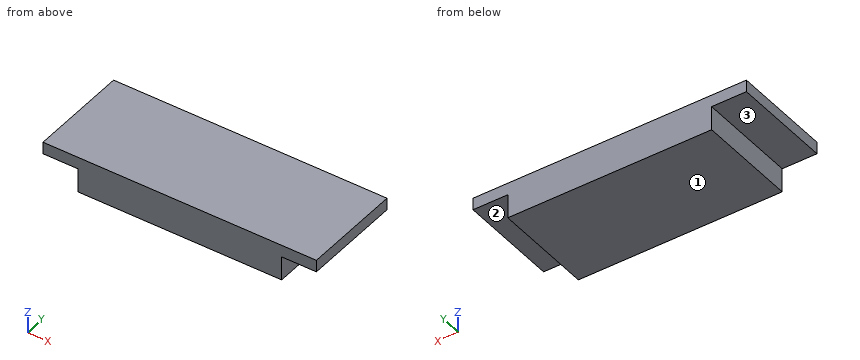
```python
from build123d import *

# Parameters (mm, degrees)
SKETCH1_W           = 57
SKETCH1_H           = 21
BOSS_EXTRUDE1_DEPTH = 2.5
SKETCH2_W           = 42.5
SKETCH2_H           = 21
BOSS_EXTRUDE2_DEPTH = 5


with BuildPart() as part:
    # Sketch1 → Boss-Extrude1 (new body)
    with BuildSketch(Plane.XY):
        Rectangle(SKETCH1_W, SKETCH1_H)
    extrude(amount=BOSS_EXTRUDE1_DEPTH)

    # Sketch2 → Boss-Extrude2 (add)
    with BuildSketch(Plane(origin=(0, 0, 0), x_dir=(-1, 0, 0), z_dir=(0, 0, -1))):
        Rectangle(SKETCH2_W, SKETCH2_H)
    extrude(amount=BOSS_EXTRUDE2_DEPTH)


solid = part.part
```
Verification items for the finished model (mm, model axes). Face numbers are marked on the shaded views. A direction names the side the tool comes from. Coordinates: 2 decimals unless noted, no trailing zeros. Write each loop counter-clockwise with the first axis right and the second up, starting at its lowest first coordinate (ties: lowest second). Pieces come first, ordered by that corner, then holes. Notation, with made-up numbers: (18.25, 37.5) - (69.25, 37.5) arc R35 cw to (69.25, 70.5) - close; hole circle Ø11 at (64, 10). An arc over 180 degrees is marked (long way). One line per question, with ' | ' between items. Start each with the question number.
1. Gauge pin test, flat ends, axial feed: P1, Ø2, axis at x = 24.5, y = 5, coming from the -Z side; P2, Ø3, axis at y = 6, z = -3.5, coming from the +X side; P3, Ø1.5, axis at y = 1.5, z = -3.5, coming from the -X side. Record the tip position at first contact, or that the pin passes through.
2. Access from +Z, -Z, +X, -X, +Y, -Y to the whole of each face (thin tool, end or side, straight path). Record for the marked faces 1, 2 and 3.
3. Section check A-A (y = 4). Enter the section's corners in (x, z), plus the area to 3 significant figures.
4. Material ranges on line 1 along X through (y, z) = (7.25, -1); line 2 along Z through (x, y) = (25, -4.25), recorded low to high.
5. Section check B-B (z = -0.75). Enter the section's corners in (x, y).
Computed values:
1) P1: z = 0 | P2: x = 21.25 | P3: x = -21.25
2) face 1: -Z, +X, -X, +Y, -Y | face 2: -Z, +X, +Y, -Y | face 3: -Z, -X, +Y, -Y
3) outline: (-28.5, 0) - (-21.25, 0) - (-21.25, -5) - (21.25, -5) - (21.25, 0) - (28.5, 0) - (28.5, 2.5) - (-28.5, 2.5) - close | area: 355 mm²
4) line 1: -21.25 to 21.25 | line 2: 0 to 2.5
5) outline: (-21.25, -10.5) - (21.25, -10.5) - (21.25, 10.5) - (-21.25, 10.5) - close
